```python
from build123d import *

# Parameters (mm, degrees)
F0_R     = 80
F1_DEPTH = 5
F2_R     = 74
F2_R_2   = 72
F3_DEPTH = 3
F4_D     = 3
F5_R     = 5


with BuildPart() as f1:
    # F0 (on Top) → F1 (new body)
    with BuildSketch(Plane.XY):
        with Locations((0, -60)):
            Circle(F0_R)
        Polygon((35, 0), (60, -25), (60, -95), (35, -120), (-35, -120), (-60, -95), (-60, -25), (-35, 0), align=None, mode=Mode.SUBTRACT)
    extrude(amount=F1_DEPTH)

    # F2 (on face) → F3 (cut)
    with BuildSketch(Plane.XY.offset(5)):
        with Locations((0, -60)):
            Circle(F2_R)
        with Locations((0, -60)):
            Circle(F2_R_2, mode=Mode.SUBTRACT)
    extrude(amount=-F3_DEPTH, mode=Mode.SUBTRACT)

    # F4 (through all)
    with Locations(Plane.XY.offset(5)):
        with Locations((-73, -60), (73, -60)):
            Hole(F4_D / 2)

    # F5
    f5_edges = [f1.edges().sort_by_distance(p)[0] for p in [
        (-35, 0, 2.5),
        (35, 0, 2.5),
        (-60, -25, 2.5),
        (60, -25, 2.5),
        (60, -95, 2.5),
        (35, -120, 2.5),
        (-35, -120, 2.5),
        (-60, -95, 2.5),
    ]]
    fillet(f5_edges, radius=F5_R)


solid = f1.part
```
Can you work these out from the model? Positions are in its coordinate system, mm. A direction names the side the tool comes from. Coordinates: 2 decimals unless noted, no trailing zeros. Order: outer loops, then holes, each group sorted by start corner. A loop starts at its lowest first (then second) coordinate and runs counter-clockwise, first axis right, second up. Notation, with made-up numbers: (-37.75, -5.75) - (5.25, -5.75) arc R35 cw to (5.25, 32.25) - close; hole circle Ø4 at (36.25, 84.5). An arc over 180 degrees is marked (long way). Answer in a Markdown table with one row per item.
1. If I drill on line 1 along X through (y, z) = (-14.5, 3.3); line 2 along Y through (x, z) = (66, 3.3); line 3 along X through (y, z) = (-90.5, 2.55), over which ranges is the centre line in solid material (lowest first)?
Reply:
| item | result |
|---|---|
| line 1 | x = -65.8 to -58.36, -55.8 to -49.5, 49.5 to 55.8, 58.36 to 65.8 |
| line 2 | y = -105.21 to -93.47, -88.77 to -31.23, -26.53 to -14.79 |
| line 3 | x = -73.96 to -67.42, -65.22 to -60, 60 to 65.22, 67.42 to 73.96 |
2. Suppose I cut it at A-A (z = 1.05). Please give me the cut outline in (x, y).
Reply:
| item | result |
|---|---|
| outline | circle Ø160 at (0, -60); hole circle Ø3 at (-73, -60); hole (-60, -92.93) arc R5 ccw to (-58.54, -96.46) - (-36.46, -118.54) arc R5 ccw to (-32.93, -120) - (32.93, -120) arc R5 ccw to (36.46, -118.54) - (58.54, -96.46) arc R5 ccw to (60, -92.93) - (60, -27.07) arc R5 ccw to (58.54, -23.54) - (36.46, -1.46) arc R5 ccw to (32.93, 0) - (-32.93, 0) arc R5 ccw to (-36.46, -1.46) - (-58.54, -23.54) arc R5 ccw to (-60, -27.07) - close; hole circle Ø3 at (73, -60) |
3. For faces 1 (the cylindrical face through (1.611, 13.982, 3.521)), 2 (the flat face through (47, -12, 2)), 3 (the flat face through (0, 6, 0)), which set-ups out of +Z, -Z, +X, -X, +Y, -Y let a thin tool reach every point of the face, with its end or its side?
Reply:
| item | result |
|---|---|
| face 1 | +Z |
| face 2 | +Z, -Z |
| face 3 | -Z, +X, -X, +Y, -Y |
4. Suppose I cut it at C-C (x = -18). Please give me the cut outline in (y, z), and give its area (3 significant figures).
Reply:
| item | result |
|---|---|
| outline | (-137.95, 0) - (-120, 0) - (-120, 5) - (-129.71, 5) - (-129.71, 2) - (-131.78, 2) - (-131.78, 5) - (-137.95, 5) - close; (0, 0) - (17.95, 0) - (17.95, 5) - (11.78, 5) - (11.78, 2) - (9.71, 2) - (9.71, 5) - (0, 5) - close |
| area | 167 mm^2 |
5. For pin 1 (1.5 mm diameter, centred on y = 2, z = 2.5, fed in from -X); pin 2 (1 mm diameter, centred on x = -50.5, z = 2.5, fed in from -Y); pin 3 (2 mm diameter, centred on x = -49, z = 3, fed in from -Y), each with a flat end and sliding along its axis, tell me the tip position at first contact or that it passes through.
Reply:
| item | result |
|---|---|
| pin 1 | stops at x = -51.46 |
| pin 2 | stops at y = -122.45 |
| pin 3 | stops at y = -124 |
6. If we mould it in two halves opening along X, with no side actions, what happens to faces 4 (the flat face through (48, -107, 2)), 5 (the cylindrical face through (-1.568, -131.983, 3.521)), 6 (the flat face through (23, -131, 5)), 7 (the cylindrical face through (36.92, -130.97, 2.46))? For each: pulls with the +X half, pulls with the -X half, needs draft (parallel to the pull), parting line crosses it, or undercut.
Reply:
| item | result |
|---|---|
| face 4 | undercut |
| face 5 | undercut |
| face 6 | needs draft |
| face 7 | parting line crosses it |
7. Suppose I cut it at B-B (y = -15.5). Please give me the cut outline in (x, z).
Reply:
| item | result |
|---|---|
| outline | (-66.48, 0) - (-50.5, 0) - (-50.5, 5) - (-56.6, 5) - (-56.6, 2) - (-59.12, 2) - (-59.12, 5) - (-66.48, 5) - close; (50.5, 0) - (66.48, 0) - (66.48, 5) - (59.12, 5) - (59.12, 2) - (56.6, 2) - (56.6, 5) - (50.5, 5) - close |
